from build123d import *

# Parameters (mm, degrees)
SKETCH1_W           = 52
SKETCH1_H           = 65
BOSS_EXTRUDE1_DEPTH = 6
FILLET1_R           = 3
SKETCH4_W           = 17
SKETCH4_H           = 3.7
CUT_EXTRUDE1_DEPTH  = 7
CUT_EXTRUDE2_DEPTH  = 7
CUT_EXTRUDE3_DEPTH  = 7


with BuildPart() as part:
    # Sketch1 → Boss-Extrude1 (new body)
    with BuildSketch(Plane(origin=(0, 0, 0), x_dir=(1, 0, 0), z_dir=(0, 1, 0))):
        Rectangle(SKETCH1_W, SKETCH1_H)
    extrude(amount=BOSS_EXTRUDE1_DEPTH)

    # Fillet1
    fillet1_edges = [part.edges().sort_by_distance(p)[0] for p in [
        (26, 3, 32.5),
        (-26, 3, 32.5),
        (-26, 3, -32.5),
        (26, 3, -32.5),
    ]]
    fillet(fillet1_edges, radius=FILLET1_R)

    # Sketch4 → Cut-Extrude1 (cut, through all)
    with BuildSketch(Plane(origin=(0, 6, 0), x_dir=(1, 0, 0), z_dir=(0, 1, 0))):
        with Locations((-12.807771524, -23.65)):
            Rectangle(SKETCH4_W, SKETCH4_H)
    cut_extrude1 = extrude(amount=-CUT_EXTRUDE1_DEPTH, mode=Mode.SUBTRACT)

    # Mirror2: Cut-Extrude1 across plane
    add(cut_extrude1.mirror(Plane(origin=(0, 0, 0), x_dir=(0, 0, 1), z_dir=(1, 0, 0))), mode=Mode.SUBTRACT)

    # Sketch5 → Cut-Extrude2 (cut, through all)
    with BuildSketch(Plane(origin=(0, 6, 0), x_dir=(1, 0, 0), z_dir=(0, 1, 0))):
        with BuildLine():
            Line((10.307771524, -13.2), (15.307771524, -13.2))
            ThreePointArc((15.307771524, -13.2), (17.707771524, -15.6), (15.307771524, -18))
            Line((15.307771524, -18), (10.307771524, -18))
            ThreePointArc((10.307771524, -18), (7.907771524, -15.6), (10.307771524, -13.2))
        make_face()
    extrude(amount=-CUT_EXTRUDE2_DEPTH, mode=Mode.SUBTRACT)

    # Sketch6 → Cut-Extrude3 (cut, through all)
    with BuildSketch(Plane(origin=(0, 6, 0), x_dir=(1, 0, 0), z_dir=(0, 1, 0))):
        with BuildLine():
            Line((-9.307771524, 25.2), (-9.307771524, 1.7))
            ThreePointArc((-9.307771524, 1.7), (-12.807771524, -1.8), (-16.307771524, 1.7))
            Line((-16.307771524, 1.7), (-16.307771524, 25.2))
            ThreePointArc((-16.307771524, 25.2), (-12.807771524, 28.7), (-9.307771524, 25.2))
        make_face()
    extrude(amount=-CUT_EXTRUDE3_DEPTH, mode=Mode.SUBTRACT)


solid = part.part
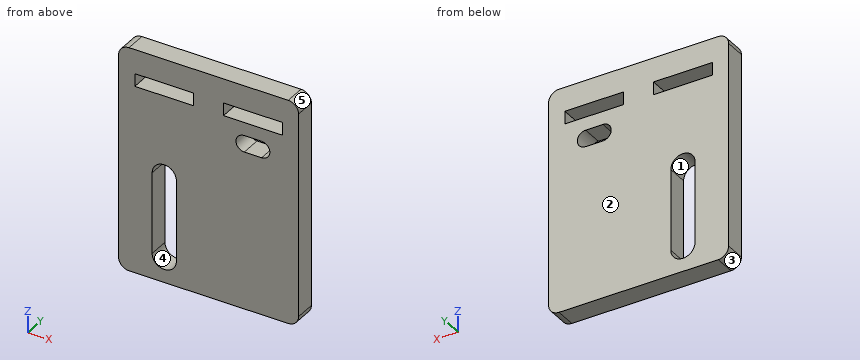
Input: part model. Units: mm. Frame: model coordinates. Face numbers are marked on the shaded views. A direction names the side the tool comes from. Coordinates: 2 decimals unless noted, no trailing zeros. Loops run counter-clockwise (first coordinate to the right, second up) from the corner with the lowest first, then second, coordinate; pieces in that order, holes last. Notation, with made-up numbers: (-24, -25) -> (35, -25) arc R21 ccw to (35, -17) -> close; hole circle Ø11 at (-4.75, 62.5). An arc over 180 degrees is marked (long way). One line per item, written item: value.
(1) Ray query, line 1 along Z through (x, y) = (-12.5, 1.75); line 2 along Z through (x, y) = (14, 5.4); line 3 along X through (y, z) = (3.6, -14). Return the intervals inside material, ascending.
Answer below:
line 1: z = -32.5 to -28.69, 1.79 to 21.8, 25.5 to 32.5
line 2: z = -32.5 to 13.2, 18 to 21.8, 25.5 to 32.5
line 3: x = -26 to -16.31, -9.31 to 26
(2) Draft query along Z for the marked faces 1, 2 and 3. Return one class per face: pulls with the +Z half, pulls with the -Z half, needs draft (parallel to the pull), parting line crosses it, or undercut.
Answer below:
face 1: undercut
face 2: needs draft
face 3: pulls with the -Z half
(3) Set-up query: the marked faces 4 and 5. Return all of +Z, -Z, +X, -X, +Y, -Y with unobstructed straight access to the full face (end or side cutting, diameter ignored); none if empty.
Answer below:
face 4: +Y, -Y
face 5: +Z, +X, +Y, -Y
(4) Cut plane C-C (x = 6.5). Output: boundary loops of the cut face in (y, z).
Answer below:
outline: (0, -32.5) -> (6, -32.5) -> (6, 21.8) -> (0, 21.8) -> close; (0, 25.5) -> (6, 25.5) -> (6, 32.5) -> (0, 32.5) -> close
(5) Cut plane B-B (z = -18.5). Output: boundary loops of the cut face in (x, y), then the cut area to 3 significant figures.
Answer below:
outline: (-26, 0) -> (-16.31, 0) -> (-16.31, 6) -> (-26, 6) -> close; (-9.31, 0) -> (26, 0) -> (26, 6) -> (-9.31, 6) -> close
area: 270 mm2
(6) Cut plane A-A (y = 5.2). Output: boundary loops of the cut face in (x, z), then the cut area to 3 significant figures.
Answer below:
outline: (-26, -29.5) arc R3 ccw to (-23, -32.5) -> (23, -32.5) arc R3 ccw to (26, -29.5) -> (26, 29.5) arc R3 ccw to (23, 32.5) -> (-23, 32.5) arc R3 ccw to (-26, 29.5) -> close; hole (-21.31, 21.8) -> (-4.31, 21.8) -> (-4.31, 25.5) -> (-21.31, 25.5) -> close; hole (-16.31, -25.2) arc R3.5 ccw to (-9.31, -25.2) -> (-9.31, -1.7) arc R3.5 ccw to (-16.31, -1.7) -> close; hole (4.31, 21.8) -> (21.31, 21.8) -> (21.31, 25.5) -> (4.31, 25.5) -> close; hole (10.31, 13.2) -> (15.31, 13.2) arc R2.4 ccw to (15.31, 18) -> (10.31, 18) arc R2.4 ccw to start
area: 3,000 mm2
